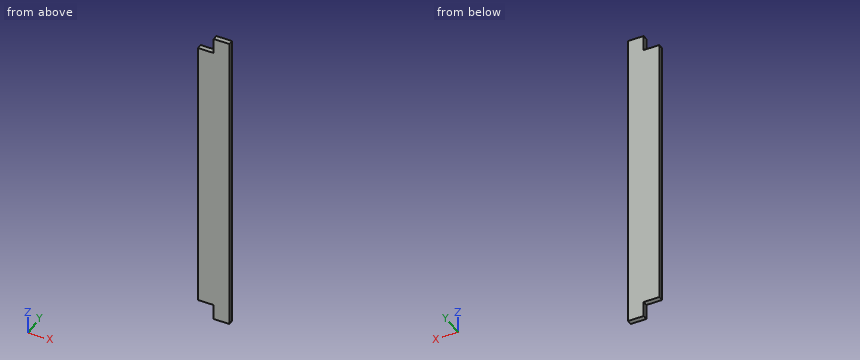
Autodesk Inventor part; units mm, degrees
ref_plane "YZ Plane" through (0, 0, 0) normal (1, 0, 0) x (0, 1, 0)
ref_plane "XZ Plane" through (0, 0, 0) normal (0, 1, 0) x (-1, 0, 0)
ref_plane "XY Plane" through (0, 0, 0) normal (0, 0, 1) x (1, 0, 0)
sketch "Sketch1" plane through (0, 0, 0) normal (0, 1, 0) x (-1, 0, 0)
  line L0 (0, 0) -> (-40, 0)
  line L1 (-40, 0) -> (-40, -400)
  line L2 (-40, -400) -> (0, -400)
  line L3 (0, -400) -> (0, 0)
  line L4 (0, 0) -> (-20, 0)
  line L5 (-20, 0) -> (-20, -20)
  line L6 (-20, -20) -> (0, -20)
  line L7 (0, -20) -> (0, 0)
  line L8 (0, -400) -> (-20, -400)
  line L9 (-20, -400) -> (-20, -380)
  line L10 (-20, -380) -> (0, -380)
  line L11 (0, -380) -> (0, -400)
  point P0 (0, -380)
  point P1 (0, -20)
  dimension "d0" = 400
  dimension "d1" = 20
  dimension "d2" = 20
  dimension "d3" = 20
  dimension "d4" = 20
  dimension "d5" = 40
extrude "Extrusion1" add sketch "Sketch1" along normal blind 6.35 contours L5 L6 L3 L10 L9 L2 L1 L0
equation "\"d0\" = base_y_dim"
equation "\"d1\" = extrusion_dim"
equation "\"d2\" = extrusion_dim"
equation "\"d3\" = extrusion_dim"
equation "\"d4\" = extrusion_dim"
equation "\"d5\" = ceiling_width"
equation "\"d6\" = top_sheet_thickness"
equation "\"base_y_dim\" = 400"
equation "\"base_thickness\" = 12.7"
equation "\"extrusion_dim\" = 20"
equation "\"top_sheet_thickness\" = 6.35"
equation "\"ceiling_width\" = 40"
properties part number "Top Sheet Metal Left"
Source: CAD feature listing. Evaluate the final solid. Frame: model axes, mm. Round coordinates to 2 decimals unless told otherwise and drop trailing zeros. Loops run counter-clockwise (first coordinate to the right, second up) from the corner with the lowest first, then second, coordinate; pieces in that order, holes last.
(1) Section query A-A (y = 4.25). Output: boundary loops of the cut face in (x, z).
From the geometry:
outline: (0, -380) - (20, -380) - (20, -400) - (40, -400) - (40, 0) - (20, 0) - (20, -20) - (0, -20) - close
(2) Section query B-B (x = 12). Output: boundary loops of the cut face in (y, z), and give its area (3 significant figures).
From the geometry:
outline: (0, -380) - (6.35, -380) - (6.35, -20) - (0, -20) - close
area: 2,290 mm2
(3) Contact query for flat-ended pins moving along their axis: pin 1 Ø1 at (x, y) = (18.5, 5) entering from +Z; pin 2 Ø1.9 at (x, y) = (13.5, 2) entering from -Z. Output: stop coordinate, or through.
From the geometry:
pin 1: stops at z = -20
pin 2: stops at z = -380
(4) Material intervals for probe 1 along Z at (x, y) = (9.5, 5), sorted ascending.
From the geometry:
probe 1: z = -380 to -20
